from build123d import *

# Parameters (mm, degrees)
F0_W       = 127
F0_H       = 127
F1_DEPTH   = 63.5
F2_W       = 42.3164
F2_H       = 31.8262
F3_DEPTH   = 25.4
F1_FACE1_W = 127
F1_FACE1_H = 127
F4_DEPTH   = 27.051
F5_W       = 42.3164
F5_H       = 31.8262
F6_DEPTH   = 57.404


with BuildPart() as f1:
    # F0 (on Front) → F1 (new body, symmetric)
    with BuildSketch(Plane.XZ):
        Rectangle(F0_W, F0_H)
    extrude(amount=F1_DEPTH, both=True)

    # F2 (on face) → F3 (cut)
    with BuildSketch(Plane.XZ.offset(63.5)):
        with Locations((-19.5812878566, -15.9131)):
            Rectangle(F2_W, F2_H)
    extrude(amount=F3_DEPTH, mode=Mode.SUBTRACT)

    # F2 (on face) + F1_face1 (on face) → F4 (join, symmetric)
    with BuildSketch(Plane.XZ.offset(63.5)):
        with Locations((-19.5812878566, -15.9131)):
            Rectangle(F2_W, F2_H)
    with BuildSketch(Plane(origin=(0, 63.5, 0), x_dir=(1, 0, 0), z_dir=(0, 1, 0))):
        Rectangle(F1_FACE1_W, F1_FACE1_H)
    extrude(amount=F4_DEPTH, both=True, dir=(0, -1, 0))

    # F5 (on face) → F6 (cut, symmetric)
    with BuildSketch(Plane(origin=(0, 90.551, 0), x_dir=(-1, 0, 0), z_dir=(0, 1, 0))):
        with Locations((19.5812878566, -15.9131)):
            Rectangle(F5_W, F5_H)
    extrude(amount=F6_DEPTH, both=True, mode=Mode.SUBTRACT)


solid = f1.part
Read the model definition and answer for the solid it produces. Units are mm, in the model's axes. A direction names the side the tool comes from. Give positions to 0.01 mm unless a question says otherwise; leave off trailing zeros. Write each loop counter-clockwise with the first axis right and the second up, starting at its lowest first coordinate (ties: lowest second). Pieces come first, ordered by that corner, then holes. Notation, with made-up numbers: (11.5, -34) - (42.5, -34) arc R22 ccw to (42.5, -15) - close; hole circle Ø2 at (31, -3). An arc over 180 degrees is marked (long way). Return JSON: item names as keys, results as strings.
Q1. A cutting plane is placed at C-C, the plane x = -6. Determine the outline of the cut face in (y, z), and give its area (3 significant figures).
Reply:
{"outline": "(-90.55, -31.83) - (-63.5, -31.83) - (-63.5, -63.5) - (90.55, -63.5) - (90.55, -31.83) - (33.15, -31.83) - (33.15, 0) - (90.55, 0) - (90.55, 63.5) - (-63.5, 63.5) - (-63.5, 0) - (-90.55, 0) - close", "area": "18,600 mm²"}
Q2. A cutting plane is placed at A-A, the plane z = -3.5. Determine the outline of the cut face in (x, y).
Reply:
{"outline": "(-63.5, -63.5) - (-40.74, -63.5) - (-40.74, -90.55) - (1.58, -90.55) - (1.58, -63.5) - (63.5, -63.5) - (63.5, 90.55) - (1.58, 90.55) - (1.58, 33.15) - (-40.74, 33.15) - (-40.74, 90.55) - (-63.5, 90.55) - close"}
Q3. For a pull along Z with two mould halves and no side action, classify faces 1 (the face through (-20, -77, 0)), 2 (the face through (13, 90.551, -1)), 3 (the face through (1.577, 62, -16)) as released by +Z, released by -Z, zero draft, split by the parting line, or undercut.
Reply:
{"face 1": "released by +Z", "face 2": "zero draft", "face 3": "undercut"}
Q4. For faces 4 (the face through (-63.5, 12, 1)), 5 (the face through (1.577, -77, -16)), 6 (the face through (-20, -77, -31.826)), 7 (the face through (-40.739, -77, -16)), 8 (the face through (-19, 62, -31.826)), determine the directions among +Z, -Z, +X, -X, +Y, -Y from which every point of the face is accessible in a straight line to the end or side of a thin tool.
Reply:
{"face 4": "+Z, -Z, -X, +Y, -Y", "face 5": "+Z, -Z, +X, -Y", "face 6": "-Z, +X, -X, -Y", "face 7": "+Z, -Z, -X, -Y", "face 8": "+Y"}
Q5. A cutting plane is placed at D-D, the plane y = -79. Determine the outline of the cut face in (x, z), and give its area (3 significant figures).
Reply:
{"outline": "(-40.74, -31.83) - (1.58, -31.83) - (1.58, 0) - (-40.74, 0) - close", "area": "1,350 mm²"}
Q6. Consider line 1 along Z through (x, y) = (-34, 36.5); line 2 along X through (y, z) = (36.5, -11); line 3 along Y through (x, z) = (49, -47). Determine where each line is inside the solid, lowest interval first. Write a range as [from, to].
Reply:
{"line 1": "[-63.5, -31.83], [0, 63.5]", "line 2": "[-63.5, -40.74], [1.58, 63.5]", "line 3": "[-63.5, 90.55]"}
Q7. A cutting plane is placed at B-B, the plane y = 75. Determine the outline of the cut face in (x, z).
Reply:
{"outline": "(-63.5, -63.5) - (63.5, -63.5) - (63.5, 63.5) - (-63.5, 63.5) - close; hole (-40.74, -31.83) - (1.58, -31.83) - (1.58, 0) - (-40.74, 0) - close"}
Q8. Given P1, Ø8, axis at y = -83.5, z = -16.5, coming from the -X side; P2, Ø13.5, axis at y = -79.5, z = -20, coming from the +X side; P3, Ø8, axis at x = -23.5, y = -71, coming from the +Z side, each flat-ended and moving along its own axis, determine where each tip first touches the part or whether it passes through.
Reply:
{"P1": "x = -40.74", "P2": "x = 1.58", "P3": "z = 0"}
